Read the model definition and answer for the solid it produces. Units are mm, in the model's axes. Coordinates: 2 decimals unless noted, no trailing zeros. Order: outer loops, then holes, each group sorted by start corner. A loop starts at its lowest first (then second) coordinate and runs counter-clockwise, first axis right, second up. Notation, with made-up numbers: (32.5, -9) - (48.5, -9) arc R18 ccw to (48.5, -1) - close; hole circle Ø11 at (41.5, 67). An arc over 180 degrees is marked (long way). Use one line per item in the form item = value.
```python
from build123d import *

# Parameters (mm, degrees)
BOSS_EXTRU_1_DEPTH      = 1.6
ESQUISSE3_R             = 1.6
ESQUISSE3_R_2           = 40
ENL_V_MAT_EXTRU_1_DEPTH = 2.6


with BuildPart() as part:
    # Esquisse1 → Boss.-Extru.1 (new body)
    with BuildSketch(Plane.XY):
        with BuildLine():
            Line((1, 0), (197, 0))
            ThreePointArc((197, 0), (197.707106781, 0.292893219), (198, 1))
            Line((198, 1), (198, 99))
            ThreePointArc((198, 99), (197.707106781, 99.707106781), (197, 100))
            Line((197, 100), (1, 100))
            ThreePointArc((1, 100), (0.292893219, 99.707106781), (0, 99))
            Line((0, 99), (0, 1))
            ThreePointArc((0, 1), (0.292893219, 0.292893219), (1, 0))
        make_face()
    extrude(amount=BOSS_EXTRU_1_DEPTH)

    # Esquisse3 → Enlèv. mat.-Extru.1 (cut, through all)
    with BuildSketch(Plane(origin=(0, 0, 0), x_dir=(-1, 0, 0), z_dir=(0, 0, -1))):
        with Locations((-179, 96)):
            Circle(ESQUISSE3_R)
        with Locations((-179, 4)):
            Circle(ESQUISSE3_R)
        with Locations((-19, 4)):
            Circle(ESQUISSE3_R)
        with Locations((-19, 96)):
            Circle(ESQUISSE3_R)
        with Locations((-100, 50)):
            Circle(ESQUISSE3_R_2)
    extrude(amount=-ENL_V_MAT_EXTRU_1_DEPTH, mode=Mode.SUBTRACT)


solid = part.part
```
(1) Section B-B, the plane x = 100 is taken. Write down the section's boundary in (y, z).
Answer list:
outline = (0, 0) - (10, 0) - (10, 1.6) - (0, 1.6) - close; (90, 0) - (100, 0) - (100, 1.6) - (90, 1.6) - close
(2) Straight lines are drawn through the part: L1, parallel to Y at x = 179, z = 1.1; L2, parallel to X at y = 51, z = 0.3; L3, parallel to Y at x = 100, z = 0.8. For each, find the intervals that lie inside material, in ascending order.
Answer list:
L1 = 0 to 2.4, 5.6 to 94.4, 97.6 to 100
L2 = 0 to 60.01, 139.99 to 198
L3 = 0 to 10, 90 to 100
(3) Section A-A, the plane y = 50 is taken. Write down the section's boundary in (x, z).
Answer list:
outline = (0, 0) - (60, 0) - (60, 1.6) - (0, 1.6) - close; (140, 0) - (198, 0) - (198, 1.6) - (140, 1.6) - close
(4) Section C-C, the plane z = 0.8 is taken. Write down the section's boundary in (x, y), then the cut area to 3 significant figures.
Answer list:
outline = (0, 1) arc R1 ccw to (1, 0) - (197, 0) arc R1 ccw to (198, 1) - (198, 99) arc R1 ccw to (197, 100) - (1, 100) arc R1 ccw to (0, 99) - close; hole circle Ø3.2 at (19, 4); hole circle Ø3.2 at (19, 96); hole circle Ø80 at (100, 50); hole circle Ø3.2 at (179, 4); hole circle Ø3.2 at (179, 96)
area = 14,700 mm2
(5) The mould has two halves that part along X. Classify faces 1 (the flat face through (76, 84, 1.6)), 2 (the cylindrical face through (63.05, 34.68, 0.79)): +X half, -X half, draft (parallel to the pull), parting line (faces both ways), or undercut.
Answer list:
face_1 = draft
face_2 = undercut
